```python
from build123d import *

# Parameters (mm, degrees)
F0_R      = 1.7272
F1_DEPTH  = 29.21
F2_W      = 46.736
F2_H      = 40.64
F3_DEPTH  = 25.4
F4_W      = 15.24
F4_H      = 6.35
F5_DEPTH  = 19.05
F6_W      = 15.24
F6_H      = 6.35
F7_DEPTH  = 19.05
F9_DEPTH  = 20.32
F11_DEPTH = 10.16
F12_SIZE2 = 0.8244325429
F12_SIZE  = 1.27
F13_W     = 25.4
F13_H     = 11.6485927218
F14_DEPTH = 101.6
F15_R     = 2.54
F16_R     = 6.35
F17_R     = 0.79502
F19_DEPTH = 5.842
F21_DEPTH = 5.842
F22_R     = 3.81
F24_DEPTH = 25.4
F26_DEPTH = 46.736
F27_R     = 2.032
F28_DEPTH = 70.6913527338


with BuildPart() as f1:
    # F0 (on Front) → F1 (new body, symmetric)
    with BuildSketch(Plane.XZ):
        Polygon((-10.16, 0), (0, 0), (0, 29.21), (0, 41.8084), (6.35, 41.8084), (6.35, 39.878), (10.16, 39.878), (12.7, 44.958), (0.0042528918, 44.958), (-10.16, 44.958), (-10.16, 37.6681894868), align=None)
        with Locations((-5.08, 5.08)):
            Circle(F0_R, mode=Mode.SUBTRACT)
        Polygon((-29.558896087, 50.2598920283), (-10.16, 37.6681894868), (-10.16, 44.958), (0.0042528918, 44.958), (-23.2167746872, 60.0306242704), align=None)
    extrude(amount=F1_DEPTH, both=True)

    # F2 (on face) → F3 (cut)
    with BuildSketch(Plane.YZ):
        with Locations((0, 20.32)):
            Rectangle(F2_W, F2_H)
    extrude(amount=-F3_DEPTH, mode=Mode.SUBTRACT)

    # F4 (on face) → F5 (cut)
    with BuildSketch(Plane(origin=(0, 29.21, 0), x_dir=(-1, 0, 0), z_dir=(0, 1, 0))):
        with Locations((-7.62, 41.783)):
            Rectangle(F4_W, F4_H)
    extrude(amount=-F5_DEPTH, mode=Mode.SUBTRACT)

    # F6 (on face) → F7 (cut)
    with BuildSketch(Plane.XZ.offset(29.21)):
        with Locations((7.62, 41.783)):
            Rectangle(F6_W, F6_H)
    extrude(amount=-F7_DEPTH, mode=Mode.SUBTRACT)

    # F8 (on face) → F9 (join)
    with BuildSketch(Plane.XZ.offset(10.16)):
        Polygon((2.8191059828, 41.8084), (0, 41.8084), (0, 40.64), align=None)
    extrude(amount=-F9_DEPTH)

    # F10 (on Front) → F11 (join, symmetric)
    with BuildSketch(Plane.XZ):
        Polygon((0.0042528918, 44.958), (12.7, 44.958), (-13.1833395176, 61.7587143563), (-16.9467400578, 55.9607838721), align=None)
    extrude(amount=F11_DEPTH, both=True)

    # F12
    f12_edges = [f1.edges().sort_by_distance(p)[0] for p in [
        (6.35, 0, 39.878),
    ]]
    f12_side = f1.faces().sort_by_distance((8.255, 0, 39.878))[0]
    chamfer(f12_edges, length=F12_SIZE, length2=F12_SIZE2, reference=f12_side)

    # F13 (on face) → F14 (join)
    with BuildSketch(Plane(origin=(-43.749584755, 0, 28.3975827839), x_dir=(0, -1, 0), z_dir=(-0.8387907858, 0, 0.5444538711))):
        with Locations((0, 31.888375289)):
            Rectangle(F13_W, F13_H)
    extrude(amount=F14_DEPTH)

    # F15
    f15_edges = [f1.edges().sort_by_distance(p)[0] for p in [
        (-13.18334, 0, 61.758714),
    ]]
    fillet(f15_edges, radius=F15_R)

    # F16
    f16_edges = [f1.edges().sort_by_distance(p)[0] for p in [
        (-26.387835, -12.7, 55.145258),
        (-26.387835, 12.7, 55.145258),
        (-111.608979, 12.7, 110.461771),
        (-111.608979, -12.7, 110.461771),
    ]]
    fillet(f16_edges, radius=F16_R)

    # F17
    f17_edges = [f1.edges().sort_by_distance(p)[0] for p in [
        (6.35, 0, 41.8084),
    ]]
    fillet(f17_edges, radius=F17_R)

    # F18 (on face) → F19 (join)
    with BuildSketch(Plane.XZ.offset(29.21)):
        Polygon((-10.16, 37.6681894868), (-29.558896087, 50.2598920283), (-10.16, 0), align=None)
    extrude(amount=-F19_DEPTH)

    # F20 (on face) → F21 (join)
    with BuildSketch(Plane(origin=(0, 29.21, 0), x_dir=(-1, 0, 0), z_dir=(0, 1, 0))):
        Polygon((10.16, 0), (29.558896087, 50.2598920283), (10.16, 37.6681894868), align=None)
    extrude(amount=-F21_DEPTH)

    # F22
    f22_edges = [f1.edges().sort_by_distance(p)[0] for p in [
        (0, -26.289, 0),
        (0, 26.289, 0),
        (-10.16, -26.289, 0),
        (-10.16, 26.289, 0),
    ]]
    fillet(f22_edges, radius=F22_R)

    # F23 (on face) → F24 (cut)
    with BuildSketch(Plane.XZ.offset(10.16)):
        with BuildLine():
            Line((-12.2835052774, 63.1450075017), (-14.5662523501, 59.6281857605))
            ThreePointArc((-14.5662523501, 59.6281857605), (-12.9643679303, 60.7296511872), (-11.0528109218, 60.3758015238))
            Line((-11.0528109218, 60.3758015238), (12.7, 44.958))
            Line((12.7, 44.958), (10.16, 39.878))
            Line((10.16, 39.878), (7.62, 39.878))
            Line((7.62, 39.878), (6.35, 40.7024325429))
            Line((6.35, 40.7024325429), (6.35, 41.01338))
            ThreePointArc((6.35, 41.01338), (6.1171440332, 41.5755440332), (5.55498, 41.8084))
            Line((5.55498, 41.8084), (2.8191059828, 41.8084))
            Line((2.8191059828, 41.8084), (0.0042528918, 40.6417626435))
            Line((0.0042528918, 40.6417626435), (0.0042528918, 37.8040261567))
            Line((0.0042528918, 37.8040261567), (17.359075731, 37.8040261567))
            Line((17.359075731, 37.8040261567), (17.359075731, 44.7986531364))
            Line((17.359075731, 44.7986531364), (-12.2835052774, 63.1450075017))
        make_face()
        with BuildLine():
            Line((-14.5662523501, 59.6281857605), (-16.9467400578, 55.9607838721))
            Line((-16.9467400578, 55.9607838721), (0.0042528918, 44.958))
            Line((0.0042528918, 44.958), (0.0042528918, 40.6417626435))
            Line((0.0042528918, 40.6417626435), (2.8191059828, 41.8084))
            Line((2.8191059828, 41.8084), (5.55498, 41.8084))
            ThreePointArc((5.55498, 41.8084), (6.1171440332, 41.5755440332), (6.35, 41.01338))
            Line((6.35, 41.01338), (6.35, 40.7024325429))
            Line((6.35, 40.7024325429), (7.62, 39.878))
            Line((7.62, 39.878), (10.16, 39.878))
            Line((10.16, 39.878), (12.7, 44.958))
            Line((12.7, 44.958), (-11.0528109218, 60.3758015238))
            ThreePointArc((-11.0528109218, 60.3758015238), (-12.9643679303, 60.7296511872), (-14.5662523501, 59.6281857605))
        make_face()
    extrude(amount=-F24_DEPTH, mode=Mode.SUBTRACT)

    # F25 (on face) → F26 (join)
    with BuildSketch(Plane.XZ.offset(-23.368)):
        Polygon((0, 40.64), (-14.738399398, 40.64), (-5.4826612016, 34.6321580255), align=None)
    extrude(amount=F26_DEPTH)

    # F27 (on face) → F28 (cut, through all)
    with BuildSketch(Plane(origin=(14.190688668, 0, 21.8623092444), x_dir=(0.8387907858, 0, -0.5444538711), z_dir=(-0.5444538711, 0, -0.8387907858))):
        with Locations((-28.5344181975, 0)):
            Circle(F27_R)
        with Locations((-38.6944181975, 0)):
            Circle(F27_R)
    extrude(amount=-F28_DEPTH, mode=Mode.SUBTRACT)


solid = f1.part
```
Work out the finished part from the listing and answer in its coordinate system (mm). A direction names the side the tool comes from. Round coordinates to 2 decimals unless told otherwise and drop trailing zeros. Write each loop counter-clockwise with the first axis right and the second up, starting at its lowest first coordinate (ties: lowest second). Pieces come first, ordered by that corner, then holes. Notation, with made-up numbers: (31, 37.5) -> (65, 37.5) arc R27 cw to (65, 60.5) -> close; hole circle Ø1 at (-3.5, 57). An arc over 180 degrees is marked (long way). Write each question's results on one line, items separated by ' | '.
1) For a pull along X with two mould halves and no side action, classify faces 1 (the cylindrical face through (-8.32, -0.09, 43.32)), 2 (the flat face through (-11, 23.368, 25)), 3 (the cylindrical face through (-27.86, -14.61, 56.2)) as +X half, -X half, draft (parallel to the pull), parting line (faces both ways), or undercut.
Findings:
face 1: undercut | face 2: draft | face 3: -X half
2) Flat-ended cylindrical pins translate along their axes: pin 1 (4 mm diameter, centred on x = -15, y = -18, fed in from -Z); pin 2 (5.5 mm diameter, centred on y = 19.5, z = 26.5, fed in from +X); pin 3 (8 mm diameter, centred on x = -45, y = 15, fed in from +Z); pin 4 (4 mm diameter, centred on x = -14.5, y = -8.5, fed in from +Z). Find the tip coordinate at first contact, or state that the pin passes through.
Findings:
pin 1: stops at z = 39.51 | pin 2: passes through | pin 3: stops at z = 76.29 | pin 4: stops at z = 55.67
3) Which of the six approach directions +Z, -Z, +X, -X, +Y, -Y give full straight-line access (tool end or side, diameter ignored) to faces 4 (the flat face through (-26.343, -24.201, 55.214)), 5 (the flat face through (-26.343, 24.059, 55.214)), 6 (the cylindrical face through (-16.4, -1.37, 48.56))?
Findings:
face 4: +Z, -X, -Y | face 5: +Z, -X, +Y | face 6: none
4) The part is cut by section C-C (z = 88). Write down the section's boundary in (x, y), and give its area (3 significant figures).
Findings:
outline: (-87.7, -12.7) -> (-66.31, -12.7) -> (-66.31, 12.7) -> (-87.7, 12.7) -> close | area: 543 mm²
5) The part is cut by section D-D (x = -91.5). Write down the section's boundary in (y, z), and give its area (3 significant figures).
Findings:
outline: (-12.7, 90.47) -> (12.7, 90.47) -> (12.7, 104.35) -> (-12.7, 104.35) -> close | area: 353 mm²
6) Consider line 1 along Z through (x, y) = (-5.08, 24.6); line 2 along Z through (x, y) = (-5, -26); line 3 along X through (y, z) = (27, 5). Determine where each line is inside the solid, lowest interval first. Write a range as [from, to].
Findings:
line 1: z = [0, 3.35], [6.81, 48.26] | line 2: z = [0, 3.35], [6.81, 48.21] | line 3: x = [-12.09, -6.81], [-3.35, 0]
7) The part is cut by section B-B (z = 10.5). Write down the section's boundary in (x, y), and give its area (3 significant figures).
Findings:
outline: (-14.21, -29.21) -> (0, -29.21) -> (0, -23.37) -> (-14.21, -23.37) -> close; (-14.21, 23.37) -> (0, 23.37) -> (0, 29.21) -> (-14.21, 29.21) -> close | area: 166 mm²
